Could you check a few things on this model? Use its own coordinates, in mm. A direction names the side the tool comes from. Give positions to 0.01 mm unless a question says otherwise; leave off trailing zeros. Write each loop counter-clockwise with the first axis right and the second up, starting at its lowest first coordinate (ties: lowest second). Pieces come first, ordered by that corner, then holes. Notation, with made-up numbers: (-6.75, -13.5) - (39.25, -13.5) arc R16 ccw to (39.25, 13.5) - close; hole circle Ø4 at (-20, 0). An arc over 180 degrees is marked (long way). Write item = value, one per line.
Autodesk Inventor part; units mm, degrees
ref_plane "YZ Plane" through (0, 0, 0) normal (1, 0, 0) x (0, 1, 0)
ref_plane "XZ Plane" through (0, 0, 0) normal (0, 1, 0) x (-1, 0, 0)
ref_plane "XY Plane" through (0, 0, 0) normal (0, 0, 1) x (1, 0, 0)
sketch "Sketch1" plane through (0, 0, 0) normal (0, 0, 1) x (1, 0, 0)
  line L0 (9.015, -16.7025) -> (6.8938, -16.7025)
  line L1 (6.8938, -16.7025) -> (6.8938, -15.94)
  arc A0 (9.015, -16.7025) -> (10.285, -15.4325) centre (9.015, -15.4325) ccw
  line L2 (6.8938, -15.94) -> (5.6348, -15.94)
  line L3 (10.285, -12.9481) -> (10.285, -15.4325)
  arc A1 (5.6348, -15.94) -> (4.06, -17.5148) centre (5.6348, -17.5148) ccw
  arc A2 (10.285, -12.9481) -> (10.024, -12.3188) centre (9.396, -12.9481) ccw
  line L4 (4.06, -17.5148) -> (4.06, -18.4252)
  line L5 (6.7733, -9.0747) -> (10.024, -12.3188)
  arc A3 (4.06, -18.4252) -> (5.6348, -20) centre (5.6348, -18.4252) ccw
  arc A4 (6.7733, -9.0747) -> (3.4312, -7.7) centre (3.4312, -12.4498) ccw
  line L6 (5.6348, -20) -> (16.825, -20)
  line L7 (-3.4312, -7.7) -> (3.4312, -7.7)
  arc A5 (16.825, -20) -> (20, -16.825) centre (16.825, -16.825) ccw
  arc A6 (-3.4312, -7.7) -> (-6.7733, -9.0747) centre (-3.4312, -12.4498) ccw
  line L8 (20, -16.825) -> (20, 16.825)
  line L9 (-10.024, -12.3188) -> (-6.7733, -9.0747)
  arc A7 (20, 16.825) -> (16.825, 20) centre (16.825, 16.825) ccw
  arc A8 (-10.024, -12.3188) -> (-10.285, -12.9481) centre (-9.396, -12.9481) ccw
  line L10 (16.825, 20) -> (5.6348, 20)
  line L11 (-10.285, -15.4325) -> (-10.285, -12.9481)
  arc A9 (5.6348, 20) -> (4.06, 18.4252) centre (5.6348, 18.4252) ccw
  arc A10 (-10.285, -15.4325) -> (-9.015, -16.7025) centre (-9.015, -15.4325) ccw
  line L12 (4.06, 18.4252) -> (4.06, 17.5148)
  line L13 (-6.8938, -16.7025) -> (-9.015, -16.7025)
  arc A11 (4.06, 17.5148) -> (5.6348, 15.94) centre (5.6348, 17.5148) ccw
  line L14 (-6.8938, -15.94) -> (-6.8938, -16.7025)
  line L15 (5.6348, 15.94) -> (6.7718, 15.94)
  line L16 (-5.6348, -15.94) -> (-6.8938, -15.94)
  line L17 (6.7718, 15.94) -> (6.7718, 16.5629)
  arc A12 (-4.06, -17.5148) -> (-5.6348, -15.94) centre (-5.6348, -17.5148) ccw
  line L18 (6.7718, 16.5629) -> (9.015, 16.5629)
  line L19 (-4.06, -18.4252) -> (-4.06, -17.5148)
  arc A13 (10.285, 15.2929) -> (9.015, 16.5629) centre (9.015, 15.2929) ccw
  arc A14 (-5.6348, -20) -> (-4.06, -18.4252) centre (-5.6348, -18.4252) ccw
  line L20 (10.285, 15.2929) -> (10.285, 12.9795)
  line L21 (-16.825, -20) -> (-5.6348, -20)
  arc A15 (10.0407, 12.3673) -> (10.285, 12.9795) centre (9.396, 12.9795) ccw
  arc A16 (-20, -16.825) -> (-16.825, -20) centre (-16.825, -16.825) ccw
  line L22 (10.0407, 12.3673) -> (6.7505, 9.0839)
  line L23 (-20, 16.825) -> (-20, -16.825)
  arc A17 (3.4141, 7.7) -> (6.7505, 9.0839) centre (3.3992, 12.4498) ccw
  arc A18 (-16.825, 20) -> (-20, 16.825) centre (-16.825, 16.825) ccw
  line L24 (3.4141, 7.7) -> (-3.4141, 7.7)
  line L25 (-5.6348, 20) -> (-16.825, 20)
  arc A19 (-6.7505, 9.0839) -> (-3.4141, 7.7) centre (-3.3992, 12.4498) ccw
  arc A20 (-4.06, 18.4252) -> (-5.6348, 20) centre (-5.6348, 18.4252) ccw
  line L26 (-6.7505, 9.0839) -> (-10.0407, 12.3673)
  line L27 (-4.06, 17.5148) -> (-4.06, 18.4252)
  arc A21 (-10.285, 12.9795) -> (-10.0407, 12.3673) centre (-9.396, 12.9795) ccw
  arc A22 (-5.6348, 15.94) -> (-4.06, 17.5148) centre (-5.6348, 17.5148) ccw
  line L28 (-10.285, 12.9795) -> (-10.285, 15.2929)
  line L29 (-6.7718, 15.94) -> (-5.6348, 15.94)
  arc A23 (-9.015, 16.5629) -> (-10.285, 15.2929) centre (-9.015, 15.2929) ccw
  line L30 (-6.7718, 16.5629) -> (-6.7718, 15.94)
  line L31 (-9.015, 16.5629) -> (-6.7718, 16.5629)
  arc A24 (11.935, -17.7218) -> (12.5645, -18.35) centre (12.57, -17.715) ccw
  line L32 (11.935, -17.7218) -> (11.935, -10.9555)
  line L33 (15.5575, -18.35) -> (12.5645, -18.35)
  arc A25 (11.935, -10.9555) -> (11.0739, -8.7045) centre (8.7609, -10.8795) ccw
  arc A26 (15.5575, -18.35) -> (18.35, -15.5575) centre (15.556, -15.556) ccw
  line L34 (11.0739, -8.7045) -> (9.1386, -6.7731)
  line L35 (18.35, 15.5575) -> (18.35, -15.5575)
  arc A27 (7.685, -3.508) -> (9.1386, -6.7731) centre (12.4322, -3.3507) ccw
  arc A28 (18.35, 15.5575) -> (15.5575, 18.35) centre (15.556, 15.556) ccw
  line L36 (7.685, -3.508) -> (7.685, 3.2977)
  line L37 (12.566, 18.35) -> (15.5575, 18.35)
  arc A29 (9.033, 6.6995) -> (7.685, 3.2977) centre (12.434, 3.3839) ccw
  arc A30 (12.566, 18.35) -> (11.935, 17.7218) centre (12.57, 17.715) ccw
  line L38 (9.033, 6.6995) -> (10.9703, 8.6329)
  line L39 (11.935, 10.9555) -> (11.935, 17.7218)
  arc A31 (10.9703, 8.6329) -> (11.935, 10.9555) centre (8.7603, 10.9125) ccw
  circle A32 centre (0, 0) radius 3.4
  arc A33 (-11.0739, -8.7045) -> (-11.935, -10.9555) centre (-8.7609, -10.8795) ccw
  line L40 (-11.935, -10.9555) -> (-11.935, -17.7218)
  line L41 (-9.1386, -6.7731) -> (-11.0739, -8.7045)
  arc A34 (-12.5645, -18.35) -> (-11.935, -17.7218) centre (-12.57, -17.715) ccw
  arc A35 (-9.1386, -6.7731) -> (-7.685, -3.508) centre (-12.4322, -3.3507) ccw
  line L42 (-12.5645, -18.35) -> (-15.5575, -18.35)
  line L43 (-7.685, 3.2977) -> (-7.685, -3.508)
  arc A36 (-18.35, -15.5575) -> (-15.5575, -18.35) centre (-15.556, -15.556) ccw
  arc A37 (-7.685, 3.2977) -> (-9.033, 6.6995) centre (-12.434, 3.3839) ccw
  line L44 (-18.35, -15.5575) -> (-18.35, 15.5575)
  line L45 (-10.9703, 8.6329) -> (-9.033, 6.6995)
  arc A38 (-15.5575, 18.35) -> (-18.35, 15.5575) centre (-15.556, 15.556) ccw
  arc A39 (-11.935, 10.9555) -> (-10.9703, 8.6329) centre (-8.7603, 10.9125) ccw
  line L46 (-15.5575, 18.35) -> (-12.566, 18.35)
  line L47 (-11.935, 17.7218) -> (-11.935, 10.9555)
  arc A40 (-11.935, 17.7218) -> (-12.566, 18.35) centre (-12.57, 17.715) ccw
extrude "Extrusion1" add sketch "Sketch1" against normal blind 100
properties part number "40-4004-BLACK-FB"
1. Thinking about a two-plate mould opening in Y: for faces 4 (the face through (-20, 0, -49)), 5 (the face through (-7.685, 0, -49)), 6 (the face through (-11, 20, -49)), which applies, pulls with the +Y half, pulls with the -Y half, needs draft (parallel to the pull), parting line crosses it, or undercut?
Filled sheet:
face_4 = needs draft
face_5 = undercut
face_6 = pulls with the +Y half
2. If we section it at B-B, the plane x = 0: Please give me the cut outline in (y, z).
Filled sheet:
outline = (-7.7, -100) - (-3.4, -100) - (-3.4, 0) - (-7.7, 0) - close; (3.4, -100) - (7.7, -100) - (7.7, 0) - (3.4, 0) - close
3. For pin 1 (3 mm diameter, centred on x = 14, y = -9.5, fed in from +Z); pin 2 (0.5 mm diameter, centred on y = -18, z = -69, fed in from +X); pin 3 (1 mm diameter, centred on x = 3, z = -72.5, fed in from +Y); pin 4 (5 mm diameter, centred on x = 3, z = -45, fed in from +Y), each with a flat end and sliding along its axis, tell me the tip position at first contact or that it passes through.
Filled sheet:
pin_1 = through
pin_2 = 19.86
pin_3 = 7.7
pin_4 = 19.99
4. If we section it at C-C, the plane z = -71: Count the separate pieces of the cut face and the enclosed holes in it, and give its area (3 significant figures).
Filled sheet:
separate_pieces = 1
enclosed_holes = 3
area = 598 mm2
5. Which directions (+Z, -Z, +X, -X, +Y, -Y) give clear straight access to the entire face, cutting with the end or side of a thin tool? Please do faces 1 (the face through (-19.05, 19.09, -49.3)), 2 (the face through (-18.35, 0, -49)), 3 (the face through (0, -7.7, -49)).
Filled sheet:
face_1 = +Z, -Z, -X, +Y
face_2 = +Z, -Z
face_3 = +Z, -Z, -Y
6. If we section it at A-A, the plane y = 0: Please give me the cut outline in (x, z) (3 decimals), and give its area (3 significant figures).
Filled sheet:
outline = (-20, -100) - (-18.35, -100) - (-18.35, 0) - (-20, 0) - close; (-7.685, -100) - (-3.4, -100) - (-3.4, 0) - (-7.685, 0) - close; (3.4, -100) - (7.685, -100) - (7.685, 0) - (3.4, 0) - close; (18.35, -100) - (20, -100) - (20, 0) - (18.35, 0) - close
area = 1,190 mm2
7. I need wall thicknesses on line 1 (X direction, y = 13.5, z = -8) (3 decimals); line 2 (X direction, y = -5.5, z = -90.5); line 3 (X direction, y = -8.5, z = -28). Which ranges of each line are inside material? Lowest first, please.
Filled sheet:
line_1 = -20 to -18.35, -11.935 to -10.285, 10.285 to 11.935, 18.35 to 20
line_2 = -20 to -18.35, -8.2 to 8.2, 18.35 to 20
line_3 = -20 to -18.35, -10.87 to -6.07, 6.07 to 10.87, 18.35 to 20
